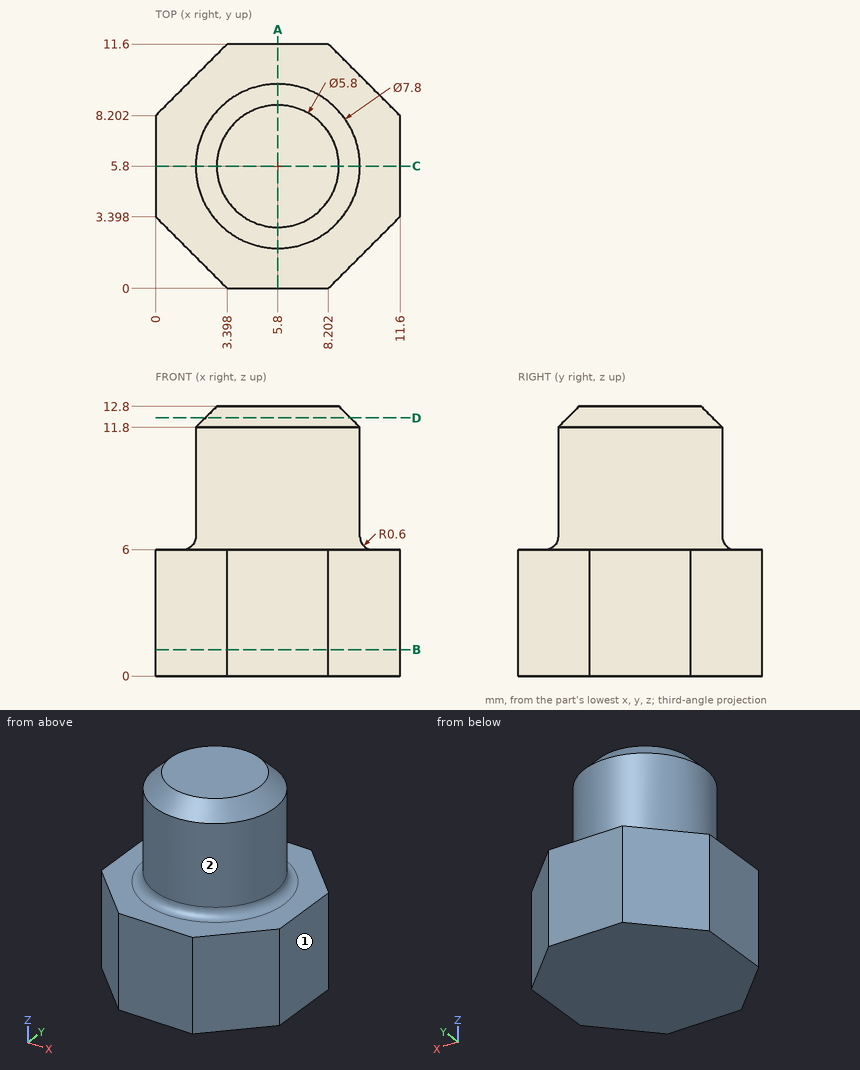
The figure shows three views and two pictorial views of one solid part (mm, origin at its lowest corner). Answer the questions. A direction names the side the tool comes from. Coordinates: 2 decimals unless noted, no trailing zeros. Loops run counter-clockwise (first coordinate to the right, second up) from the corner with the lowest first, then second, coordinate; pieces in that order, holes last.
(1) Consider line 1 along Z through (x, y) = (7.25, 10.25); line 2 along X through (y, z) = (5.25, 6.25) (1 decimal); line 3 along Y through (x, z) = (3.75, 10.25). Determine where each line is inside the solid, lowest interval first.
Solution:
line 1: z = 0 to 6
line 2: x = 1.8 to 9.8
line 3: y = 2.48 to 9.12
(2) The part is cut by section B-B (z = 1.25). Determine the outline of the cut face in (x, y).
Solution:
outline: (0, 3.4) - (3.4, 0) - (8.2, 0) - (11.6, 3.4) - (11.6, 8.2) - (8.2, 11.6) - (3.4, 11.6) - (0, 8.2) - close
(3) The part is cut by section A-A (x = 5.8). Determine the outline of the cut face in (y, z).
Solution:
outline: (0, 0) - (11.6, 0) - (11.6, 6) - (10.3, 6) arc R0.6 cw to (9.7, 6.6) - (9.7, 11.8) - (8.7, 12.8) - (2.9, 12.8) - (1.9, 11.8) - (1.9, 6.6) arc R0.6 cw to (1.3, 6) - (0, 6) - close
(4) Flat-ended cylindrical pins translate along their axes: pin 1 Ø1 at (x, y) = (1.5, 8) entering from +Z (1 decimal); pin 2 Ø5 at (x, y) = (1.5, 2) entering from +Z; pin 3 Ø1.5 at (y, z) = (10, 2) entering from +X. Find the tip coordinate at first contact, or state that the pin passes through.
Solution:
pin 1: stops at z = 6
pin 2: stops at z = 12.46
pin 3: stops at x = 10.55
(5) A tool of negligible diameter and unlimited length cuts with its end or side. For the marked faces 1 and 2, from which of +Z, -Z, +X, -X, +Y, -Y can it reach the whole face along a straight path? Write none if from no direction.
Solution:
face 1: +Z, -Z, +X, +Y, -Y
face 2: +Z
(6) The part is cut by section D-D (z = 12.25). Determine the outline of the cut face in (x, y).
Solution:
outline: circle Ø6.9 at (5.8, 5.8)
